CAD build for the part. Positions are in the model's coordinates, mm. A direction names the side the tool comes from. Round coordinates to 2 decimals unless told otherwise and drop trailing zeros. Loops run counter-clockwise (first coordinate to the right, second up) from the corner with the lowest first, then second, coordinate; pieces in that order, holes last.
```python
from build123d import *

# Parameters (mm, degrees)
SKETCH1_W           = 145
SKETCH1_H           = 20
BOSS_EXTRUDE1_DEPTH = 3
SKETCH2_R           = 3.5
SKETCH2_R_2         = 6
SKETCH2_W           = 26
SKETCH2_H           = 12
CUT_EXTRUDE1_DEPTH  = 4


with BuildPart() as part:
    # Sketch1 → Boss-Extrude1 (new body)
    with BuildSketch(Plane.XY):
        with Locations((72.5, 10)):
            Rectangle(SKETCH1_W, SKETCH1_H)
    extrude(amount=BOSS_EXTRUDE1_DEPTH)

    # Sketch2 → Cut-Extrude1 (cut, through all)
    with BuildSketch(Plane.XY.offset(3)):
        with Locations((87, 10)):
            Circle(SKETCH2_R)
        with Locations((112, 10)):
            Circle(SKETCH2_R_2)
        with Locations((30, 10)):
            Rectangle(SKETCH2_W, SKETCH2_H)
    extrude(amount=-CUT_EXTRUDE1_DEPTH, mode=Mode.SUBTRACT)


solid = part.part
```
Item 1: Probe line 1 (Y direction, x = 112, z = 0.6); line 2 (X direction, y = 8.5, z = 1); line 3 (X direction, y = 10.75, z = 1.6). List the from-to ranges inside material, lowest first.
Answers follow:
line 1: y = 0 to 4, 16 to 20
line 2: x = 0 to 17, 43 to 83.84, 90.16 to 106.19, 117.81 to 145
line 3: x = 0 to 17, 43 to 83.58, 90.42 to 106.05, 117.95 to 145
Item 2: 3-axis set-ups, long thin cutter, end or side, ignore diameter. For faces 1 (the flat face through (17, 10, 2)), 2 (the flat face through (71, 10, 0)): which of +Z, -Z, +X, -X, +Y, -Y reach the whole face in a straight line?
Answers follow:
face 1: +Z, -Z
face 2: -Z, +X, -X, +Y, -Y
Item 3: Two-plate mould, pull along X, no slides. Class faces 3 (the flat face through (71, 0, 1)), 4 (the flat face through (145, 10, 1)), 5 (the flat face through (43, 10, 2)): released by +X, released by -X, zero draft, split by the parting line, or undercut.
Answers follow:
face 3: zero draft
face 4: released by +X
face 5: undercut
Item 4: Cut at A-A, the plane x = 112. Give the cut face in (y, z), plus the area to 3 significant figures.
Answers follow:
outline: (0, 0) - (4, 0) - (4, 3) - (0, 3) - close; (16, 0) - (20, 0) - (20, 3) - (16, 3) - close
area: 24.0 mm2
Item 5: Cut at D-D, the plane x = 87. Give the cut face in (y, z).
Answers follow:
outline: (0, 0) - (6.5, 0) - (6.5, 3) - (0, 3) - close; (13.5, 0) - (20, 0) - (20, 3) - (13.5, 3) - close
Item 6: Cut at C-C, the plane z = 0.9. Give the cut face in (x, y).
Answers follow:
outline: (0, 0) - (145, 0) - (145, 20) - (0, 20) - close; hole (17, 4) - (43, 4) - (43, 16) - (17, 16) - close; hole circle Ø7 at (87, 10); hole circle Ø12 at (112, 10)
Item 7: Cut at B-B, the plane y = 10. Give the cut face in (x, z), plus the area to 3 significant figures.
Answers follow:
outline: (0, 0) - (17, 0) - (17, 3) - (0, 3) - close; (43, 0) - (83.5, 0) - (83.5, 3) - (43, 3) - close; (90.5, 0) - (106, 0) - (106, 3) - (90.5, 3) - close; (118, 0) - (145, 0) - (145, 3) - (118, 3) - close
area: 300 mm2
